Could you check a few things on this model? Use its own coordinates, in mm. A direction names the side the tool comes from. Coordinates: 2 decimals unless noted, no trailing zeros. Loops run counter-clockwise (first coordinate to the right, second up) from the corner with the lowest first, then second, coordinate; pieces in that order, holes last. Notation, with made-up numbers: (68, -23.75) - (96, -23.75) arc R17 ccw to (96, -1.75) - close; hole circle Ø11 at (44.5, 16). An arc over 180 degrees is marked (long way). One line per question, with ' | ' between items. Start each with the question number.
1. I want a section at B-B, the plane y = 8.75. Write out the boundary of the cut face in (x, z), then the cut area to 3 significant figures.
2. Which directions (+Z, -Z, +X, -X, +Y, -Y) give clear straight access to the entire face, cutting with the end or side of a thin tool? Please do faces 4 (the cylindrical face through (11.714, 4.799, 2.465)), 5 (the cylindrical face through (-10.65, 6.86, 2.46)), 6 (the cylindrical face through (5.73, -11.09, 2.46)).
3. We'd pull the mould along X, two halves only. Please class faces 1 (the cylindrical face through (-3.406, -11.99, 2.465)), 2 (the cylindrical face through (-9.283, 8.729, 2.465)), 3 (the cylindrical face through (12.43, -2.12, 2.46)): pulls with the +X half, pulls with the -X half, needs draft (parallel to the pull), parting line crosses it, or undercut.
4. I want a section at A-A, the plane y = 12.25. Write out the boundary of the cut face in (x, z).
5. Please list where these lines run through material, in increasing order: L1, parallel to Y at x = 0, z = 1.9 (3 decimals); L2, parallel to Y at x = -11, z = 3.4; L3, parallel to Y at x = -12.5, z = 1.35. Write a range as [from, to].
6. I'm going to push a flat-ended pin straight in: P1, Ø2, axis at x = -0.5, y = 9, coming from the -Z side. Where does the tip first touch, or does it pass through?
from build123d import *

# Parameters (mm, degrees)
SKETCH_1_R               = 10.875
EXTRUDE_1_DEPTH          = 5
EXTRUDE_2_DEPTH          = 5
FILLET_1_R               = 0.35
PATTERN_CIRCULAR_1_DEPTH = 5
CUT_EXTRUDE_1_REACH      = 22.572
SKETCH_2_R               = 7.5


# Read off the part's stored shape, not the designer's step: 원형 패턴1
with BuildPart() as part:
    # 스케치1 → 보스-돌출1 (new body)
    with BuildSketch(Plane.XY):
        Circle(SKETCH_1_R)
    extrude(amount=EXTRUDE_1_DEPTH)

    # 스케치1<3> → 보스-돌출2 (add)
    with BuildSketch(Plane.XY):
        with BuildLine():
            ThreePointArc((1.5525, 10.763613183), (1.216970842, 12.576974386), (0.4275, 14.243586057))
            ThreePointArc((0.4275, 14.243586057), (0, 14.25), (-0.4275, 14.243586057))
            ThreePointArc((-0.4275, 14.243586057), (-1.216970842, 12.576974386), (-1.5525, 10.763613183))
            ThreePointArc((-1.5525, 10.763613183), (0, 10.875), (1.5525, 10.763613183))
        make_face()
    extrude(amount=EXTRUDE_2_DEPTH)

    # 필렛1
    fillet_1_edges = [part.edges().sort_by_distance(p)[0] for p in [
        (-1.5525, 10.763613183, 2.5),
        (1.5525, 10.763613183, 2.5),
    ]]
    fillet(fillet_1_edges, radius=FILLET_1_R)

    # 원형 패턴1 outline → 원형 패턴1 (add)
    with BuildSketch(Plane.XY):
        with BuildLine():
            ThreePointArc((2.084837088, 10.673288121), (3.842906104, 10.173381821), (5.492422476, 9.386102511))
            ThreePointArc((5.492422476, 9.386102511), (5.344646109, 9.557145045), (5.332233471, 9.782842475))
            ThreePointArc((5.332233471, 9.782842475), (5.593355494, 11.4564781), (5.452236305, 13.144472855))
            ThreePointArc((5.452236305, 13.144472855), (5.055921411, 13.304884491), (4.654972549, 13.453334479))
            ThreePointArc((4.654972549, 13.453334479), (3.403689946, 12.289385973), (2.465385752, 10.861075951))
            ThreePointArc((2.465385752, 10.861075951), (2.306817266, 10.702930709), (2.084837088, 10.673288121))
        make_face()
        with BuildLine():
            ThreePointArc((5.736195698, 9.2391387), (7.199095251, 8.150990895), (8.459646862, 6.833739823))
            ThreePointArc((8.459646862, 6.833739823), (8.381997736, 7.045900933), (8.450146114, 7.261301773))
            ThreePointArc((8.450146114, 7.261301773), (9.274201483, 8.707038787), (9.740617886, 10.304436202))
            ThreePointArc((9.740617886, 10.304436202), (9.42901262, 10.597181051), (9.108765262, 10.880445977))
            ThreePointArc((9.108765262, 10.880445977), (7.536352291, 10.255192371), (6.155612256, 9.27693802))
            ThreePointArc((6.155612256, 9.27693802), (5.952224819, 9.187903085), (5.736195698, 9.2391387))
        make_face()
        with BuildLine():
            ThreePointArc((8.656847778, 6.582143386), (9.631277253, 5.050160738), (10.337248772, 3.377412148))
            ThreePointArc((10.337248772, 3.377412148), (10.339832595, 3.602419922), (10.478866532, 3.779351375))
            ThreePointArc((10.478866532, 3.779351375), (11.729603042, 4.815098477), (12.713475046, 6.107038785))
            ThreePointArc((12.713475046, 6.107038785), (12.528663426, 6.492580033), (12.332368752, 6.872403399))
            ThreePointArc((12.332368752, 6.872403399), (10.671238348, 6.86130469), (9.057778331, 6.466052652))
            ThreePointArc((9.057778331, 6.466052652), (8.838113972, 6.457792134), (8.656847778, 6.582143386))
        make_face()
        with BuildLine():
            ThreePointArc((10.44566348, 3.025514743), (10.802249116, 1.255802147), (10.861158072, -0.548516485))
            ThreePointArc((10.861158072, -0.548516485), (10.943077602, -0.34062274), (11.134084318, -0.224661311))
            ThreePointArc((11.134084318, -0.224661311), (12.626546762, 0.289328326), (13.969306954, 1.119162384))
            ThreePointArc((13.969306954, 1.119162384), (13.936248813, 1.545430549), (13.890417506, 1.970515105))
            ThreePointArc((13.890417506, 1.970515105), (12.377771936, 2.549980076), (10.773358461, 2.772990553))
            ThreePointArc((10.773358461, 2.772990553), (10.568207288, 2.845653785), (10.44566348, 3.025514743))
        make_face()
        with BuildLine():
            ThreePointArc((10.831434222, -0.972449329), (10.524388312, -2.739137757), (9.931200049, -4.431353133))
            ThreePointArc((9.931200049, -4.431353133), (10.080749628, -4.26807205), (10.298365111, -4.227215102))
            ThreePointArc((10.298365111, -4.227215102), (11.831510548, -4.270865326), (13.338506551, -3.985552654))
            ThreePointArc((13.338506551, -3.985552654), (13.461666574, -3.57612745), (13.572488407, -3.163191729))
            ThreePointArc((13.572488407, -3.163191729), (12.409057254, -2.103647039), (11.041512467, -1.325168872))
            ThreePointArc((11.041512467, -1.325168872), (10.879326869, -1.182845296), (10.831434222, -0.972449329))
        make_face()
        with BuildLine():
            ThreePointArc((9.724818044, -4.867600951), (8.799895988, -6.389636578), (7.638946645, -7.74029193))
            ThreePointArc((7.638946645, -7.74029193), (7.835322049, -7.642919348), (8.051101932, -7.68143897))
            ThreePointArc((8.051101932, -7.68143897), (9.434573038, -8.250170344), (10.906266927, -8.517686277))
            ThreePointArc((10.906266927, -8.517686277), (11.169011671, -8.180399177), (11.421519541, -7.835381548))
            ThreePointArc((11.421519541, -7.835381548), (10.743744256, -6.465085659), (9.78938361, -5.27081353))
            ThreePointArc((9.78938361, -5.27081353), (9.692203368, -5.079599132), (9.724818044, -4.867600951))
        make_face()
        with BuildLine():
            ThreePointArc((7.250855805, -8.104980882), (5.839114845, -9.174440736), (4.272503154, -10.000567074))
            ThreePointArc((4.272503154, -10.000567074), (4.488726043, -9.981391229), (4.674670149, -10.09339498))
            ThreePointArc((4.674670149, -10.09339498), (5.746046713, -11.099844355), (7.00107552, -11.865148727))
            ThreePointArc((7.00107552, -11.865148727), (7.367919852, -11.645552222), (7.728011172, -11.415049228))
            ThreePointArc((7.728011172, -11.415049228), (7.598229184, -9.929070664), (7.162058655, -8.502630716))
            ThreePointArc((7.162058655, -8.502630716), (7.142629708, -8.289552802), (7.250855805, -8.104980882))
        make_face()
        with BuildLine():
            ThreePointArc((3.745858716, -10.209513577), (2.04453627, -10.681081239), (0.289330355, -10.871150489))
            ThreePointArc((0.289330355, -10.871150489), (0.495925275, -10.93192564), (0.627834307, -11.102146342))
            ThreePointArc((0.627834307, -11.102146342), (1.261761796, -12.417365945), (2.150350071, -13.57584665))
            ThreePointArc((2.150350071, -13.57584665), (2.57174963, -13.503598465), (2.990792071, -13.418740812))
            ThreePointArc((2.990792071, -13.418740812), (3.40225572, -12.010026536), (3.516526006, -10.546906395))
            ThreePointArc((3.516526006, -10.546906395), (3.576953157, -10.341342504), (3.745858716, -10.209513577))
        make_face()
        with BuildLine():
            ThreePointArc((-0.289330355, -10.871150489), (-2.04453627, -10.681081239), (-3.745858716, -10.209513577))
            ThreePointArc((-3.745858716, -10.209513577), (-3.576953157, -10.341342504), (-3.516526006, -10.546906395))
            ThreePointArc((-3.516526006, -10.546906395), (-3.40225572, -12.010026536), (-2.990792071, -13.418740812))
            ThreePointArc((-2.990792071, -13.418740812), (-2.57174963, -13.503598465), (-2.150350071, -13.57584665))
            ThreePointArc((-2.150350071, -13.57584665), (-1.261761796, -12.417365945), (-0.627834307, -11.102146342))
            ThreePointArc((-0.627834307, -11.102146342), (-0.495925275, -10.93192564), (-0.289330355, -10.871150489))
        make_face()
        with BuildLine():
            ThreePointArc((-4.272503154, -10.000567074), (-5.839114845, -9.174440736), (-7.250855805, -8.104980882))
            ThreePointArc((-7.250855805, -8.104980882), (-7.142629708, -8.289552802), (-7.162058655, -8.502630716))
            ThreePointArc((-7.162058655, -8.502630716), (-7.598229184, -9.929070664), (-7.728011172, -11.415049228))
            ThreePointArc((-7.728011172, -11.415049228), (-7.367919852, -11.645552222), (-7.00107552, -11.865148727))
            ThreePointArc((-7.00107552, -11.865148727), (-5.746046713, -11.099844355), (-4.674670149, -10.09339498))
            ThreePointArc((-4.674670149, -10.09339498), (-4.488726043, -9.981391229), (-4.272503154, -10.000567074))
        make_face()
        with BuildLine():
            ThreePointArc((-7.638946645, -7.74029193), (-8.799895988, -6.389636578), (-9.724818044, -4.867600951))
            ThreePointArc((-9.724818044, -4.867600951), (-9.692203368, -5.079599132), (-9.78938361, -5.27081353))
            ThreePointArc((-9.78938361, -5.27081353), (-10.743744256, -6.465085659), (-11.421519541, -7.835381548))
            ThreePointArc((-11.421519541, -7.835381548), (-11.169011671, -8.180399177), (-10.906266927, -8.517686277))
            ThreePointArc((-10.906266927, -8.517686277), (-9.434573038, -8.250170344), (-8.051101932, -7.68143897))
            ThreePointArc((-8.051101932, -7.68143897), (-7.835322049, -7.642919348), (-7.638946645, -7.74029193))
        make_face()
        with BuildLine():
            ThreePointArc((-9.931200049, -4.431353133), (-10.524388312, -2.739137757), (-10.831434222, -0.972449329))
            ThreePointArc((-10.831434222, -0.972449329), (-10.879326869, -1.182845296), (-11.041512467, -1.325168872))
            ThreePointArc((-11.041512467, -1.325168872), (-12.409057254, -2.103647039), (-13.572488407, -3.163191729))
            ThreePointArc((-13.572488407, -3.163191729), (-13.461666574, -3.57612745), (-13.338506551, -3.985552654))
            ThreePointArc((-13.338506551, -3.985552654), (-11.831510548, -4.270865326), (-10.298365111, -4.227215102))
            ThreePointArc((-10.298365111, -4.227215102), (-10.080749628, -4.26807205), (-9.931200049, -4.431353133))
        make_face()
        with BuildLine():
            ThreePointArc((-10.861158072, -0.548516485), (-10.802249116, 1.255802147), (-10.44566348, 3.025514743))
            ThreePointArc((-10.44566348, 3.025514743), (-10.568207288, 2.845653785), (-10.773358461, 2.772990553))
            ThreePointArc((-10.773358461, 2.772990553), (-12.377771936, 2.549980076), (-13.890417506, 1.970515105))
            ThreePointArc((-13.890417506, 1.970515105), (-13.936248813, 1.545430549), (-13.969306954, 1.119162384))
            ThreePointArc((-13.969306954, 1.119162384), (-12.626546762, 0.289328326), (-11.134084318, -0.224661311))
            ThreePointArc((-11.134084318, -0.224661311), (-10.943077602, -0.34062274), (-10.861158072, -0.548516485))
        make_face()
        with BuildLine():
            ThreePointArc((-10.337248772, 3.377412148), (-9.631277253, 5.050160738), (-8.656847778, 6.582143386))
            ThreePointArc((-8.656847778, 6.582143386), (-8.838113972, 6.457792134), (-9.057778331, 6.466052652))
            ThreePointArc((-9.057778331, 6.466052652), (-10.671238348, 6.86130469), (-12.332368752, 6.872403399))
            ThreePointArc((-12.332368752, 6.872403399), (-12.528663426, 6.492580033), (-12.713475046, 6.107038785))
            ThreePointArc((-12.713475046, 6.107038785), (-11.729603042, 4.815098477), (-10.478866532, 3.779351375))
            ThreePointArc((-10.478866532, 3.779351375), (-10.339832595, 3.602419922), (-10.337248772, 3.377412148))
        make_face()
        with BuildLine():
            ThreePointArc((-8.459646862, 6.833739823), (-7.199095251, 8.150990895), (-5.736195698, 9.2391387))
            ThreePointArc((-5.736195698, 9.2391387), (-5.952224819, 9.187903085), (-6.155612256, 9.27693802))
            ThreePointArc((-6.155612256, 9.27693802), (-7.536352291, 10.255192371), (-9.108765262, 10.880445977))
            ThreePointArc((-9.108765262, 10.880445977), (-9.42901262, 10.597181051), (-9.740617886, 10.304436202))
            ThreePointArc((-9.740617886, 10.304436202), (-9.274201483, 8.707038787), (-8.450146114, 7.261301773))
            ThreePointArc((-8.450146114, 7.261301773), (-8.381997736, 7.045900933), (-8.459646862, 6.833739823))
        make_face()
        with BuildLine():
            ThreePointArc((-2.465385752, 10.861075951), (-3.403689946, 12.289385973), (-4.654972549, 13.453334479))
            ThreePointArc((-4.654972549, 13.453334479), (-5.055921411, 13.304884491), (-5.452236305, 13.144472855))
            ThreePointArc((-5.452236305, 13.144472855), (-5.593355494, 11.4564781), (-5.332233471, 9.782842475))
            ThreePointArc((-5.332233471, 9.782842475), (-5.344646109, 9.557145045), (-5.492422476, 9.386102511))
            ThreePointArc((-5.492422476, 9.386102511), (-3.842906104, 10.173381821), (-2.084837088, 10.673288121))
            ThreePointArc((-2.084837088, 10.673288121), (-2.306817266, 10.702930709), (-2.465385752, 10.861075951))
        make_face()
    extrude(amount=PATTERN_CIRCULAR_1_DEPTH)

    # 스케치2 → 컷-돌출1 (cut, up to next)
    with BuildSketch(Plane.XY.offset(5), mode=Mode.PRIVATE) as cut_extrude_1_sk1:
        Circle(SKETCH_2_R)
    cut_extrude_1_tool1 = extrude(cut_extrude_1_sk1.sketch, amount=-CUT_EXTRUDE_1_REACH, mode=Mode.PRIVATE) & part.part
    add(cut_extrude_1_tool1.solids().sort_by_distance((0, 0, 5))[0], mode=Mode.SUBTRACT)


solid = part.part
Results are:
1) outline: (-9.29, 0) - (9.29, 0) - (9.29, 5) - (-9.29, 5) - close | area: 92.9 mm2
2) face 4: +Z, -Z, +X | face 5: +Z, -Z | face 6: +Z, -Z, -Y
3) face 1: undercut | face 2: pulls with the -X half | face 3: pulls with the +X half
4) outline: (-5.58, 0) - (-3.37, 0) - (-3.37, 5) - (-5.58, 5) - close; (-1.31, 0) - (1.31, 0) - (1.31, 5) - (-1.31, 5) - close; (3.37, 0) - (5.58, 0) - (5.58, 5) - (3.37, 5) - close
5) L1: y = [-10.875, -7.5], [7.5, 14.25] | L2: y = [-8.4, -6.9], [-4.29, -1.3], [-0.29, 2.76], [4.15, 6.89] | L3: y = [-4.19, -2.17], [0.23, 2.52], [5.77, 6.55]
6) P1: stops at z = 0
